Input: dimensioned drawing with shaded views. Units: mm. Origin: part minimum x, y, z. A direction names the side the tool comes from. Coordinates: 2 decimals unless noted, no trailing zeros. Order: outer loops, then holes, each group sorted by start corner. A loop starts at its lowest first (then second) coordinate and runs counter-clockwise, first axis right, second up. Notation, with made-up numbers: (-3, -11) - (21, -11) arc R26 ccw to (21, 26) - close; hole circle Ø11 at (31.5, 36.5). An arc over 180 degrees is marked (long way). Use one line per item in the form item = value. Start each with the question number.
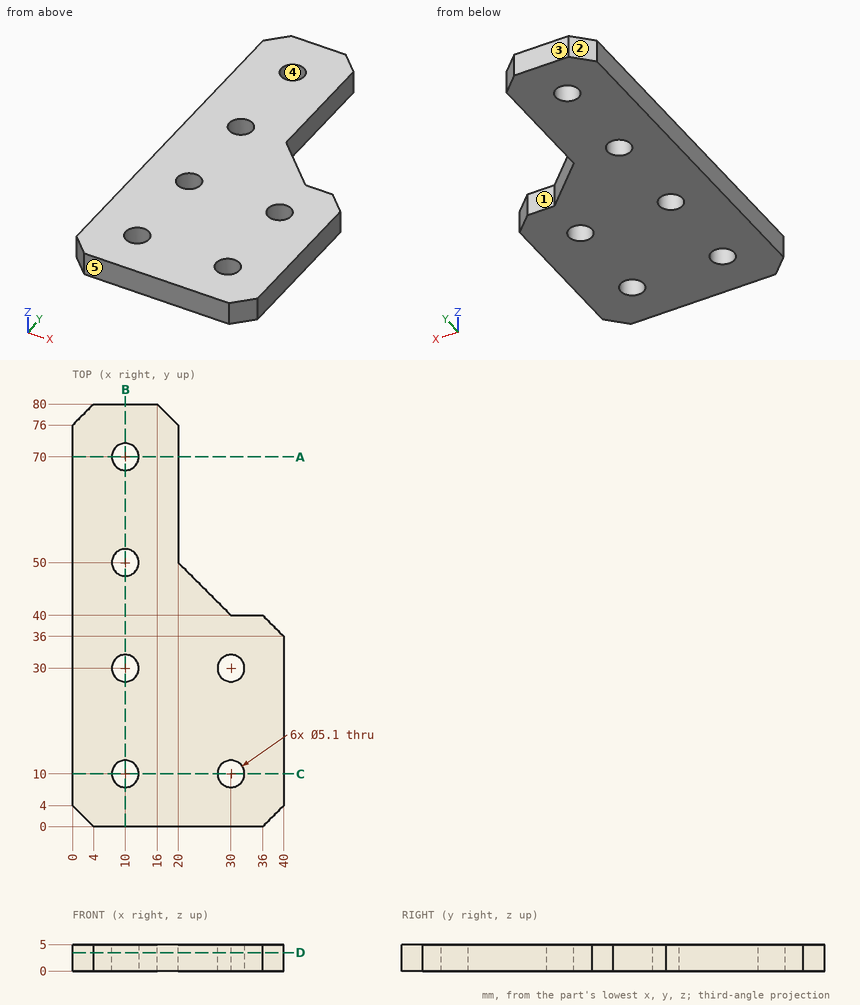
(1) Cut plane D-D on z = 3.5. Return the cut outline in (x, y).
(2) Cut plane A-A on y = 70. Return the cut outline in (x, z).
(3) Cut plane B-B on x = 10. Return the cut outline in (y, z).
(4) Contact query for a flat-ended pin moving along its axis: pin 1 Ø1.5 at (y, z) = (66, 3.5) entering from +X. Output: stop coordinate, or through.
(5) Set-up query: the marked faces 1 and 2. Return all of +Z, -Z, +X, -X, +Y, -Y with unobstructed straight access to the full face (end or side cutting, diameter ignored); none if empty.
(6) Cut plane C-C on y = 10. Return the cut outline in (x, z), plus the area to 3 significant figures.
(7) Draft query along Y for the marked faces 3, 4 and 5. Return one class per face: released by +Y, released by -Y, zero draft, split by the parting line, or undercut.
(8) Material intervals for L1, parallel to Y at x = 10, z = 1.5; L2, parallel to Y at x = 29.5, z = 1.3; L3, parallel to Y at x = 11, z = 4.7, sorted ascending. Write a range as from..to.
Check sheet entries:
q1.outline = (0, 4) - (4, 0) - (36, 0) - (40, 4) - (40, 36) - (36, 40) - (30, 40) - (20, 50) - (20, 76) - (16, 80) - (4, 80) - (0, 76) - close; hole circle Ø5.1 at (10, 10); hole circle Ø5.1 at (10, 30); hole circle Ø5.1 at (10, 50); hole circle Ø5.1 at (10, 70); hole circle Ø5.1 at (30, 10); hole circle Ø5.1 at (30, 30)
q2.outline = (0, 0) - (7.45, 0) - (7.45, 5) - (0, 5) - close; (12.55, 0) - (20, 0) - (20, 5) - (12.55, 5) - close
q3.outline = (0, 0) - (7.45, 0) - (7.45, 5) - (0, 5) - close; (12.55, 0) - (27.45, 0) - (27.45, 5) - (12.55, 5) - close; (32.55, 0) - (47.45, 0) - (47.45, 5) - (32.55, 5) - close; (52.55, 0) - (67.45, 0) - (67.45, 5) - (52.55, 5) - close; (72.55, 0) - (80, 0) - (80, 5) - (72.55, 5) - close
q4.pin_1 = 20
q5.face_1 = +Z, -Z, +X, +Y
q5.face_2 = +Z, -Z, -X, +Y
q6.outline = (0, 0) - (7.45, 0) - (7.45, 5) - (0, 5) - close; (12.55, 0) - (27.45, 0) - (27.45, 5) - (12.55, 5) - close; (32.55, 0) - (40, 0) - (40, 5) - (32.55, 5) - close
q6.area = 149 mm^2
q7.face_3 = released by +Y
q7.face_4 = undercut
q7.face_5 = released by -Y
q8.L1 = 0..7.45, 12.55..27.45, 32.55..47.45, 52.55..67.45, 72.55..80
q8.L2 = 0..7.5, 12.5..27.5, 32.5..40.5
q8.L3 = 0..7.65, 12.35..27.65, 32.35..47.65, 52.35..67.65, 72.35..80
